Study the drawing (mm; zero at the part's minimum x, y, z) and answer. A direction names the side the tool comes from. Give positions to 0.01 mm unless a question says otherwise; leave off trailing zeros. Order: outer loops, then holes, each group sorted by start corner. A loop starts at its lowest first (then second) coordinate and runs counter-clockwise, first axis right, second up. Notation, with made-up numbers: (9.5, 43) - (23.5, 43) arc R12 ccw to (23.5, 51) - close; hole circle Ø2 at (18.5, -39). An arc over 180 degrees is marked (long way). Write each question's results on one line, items separated by ' | '. Start each with the question number.
Q1. Find section C-C on y = 48. Give the vertices of the cut face in (x, z).
Q2. A tool of negligible diameter and unlimited length cuts with its end or side. For the marked faces 4 and 5, from which of +Z, -Z, +X, -X, +Y, -Y can it reach the whole face along a straight path? Write none if from no direction.
Q3. Find section A-A on z = 48. Give the vertices of the cut face in (x, y).
Q4. Flat-ended cylindrical pins translate along their axes: P1, Ø3, axis at y = 71.5, z = 22, coming from the -X side; P2, Ø2, axis at x = 6.5, z = 35.5, coming from the +Y side; P3, Ø3, axis at x = 5, z = 37, coming from the +Y side. Find the tip coordinate at first contact, or state that the pin passes through.
Q5. For a pull along Z with two mould halves and no side action, classify the marked faces 1, 2 and 3 as +Z half, -Z half, draft (parallel to the pull), parting line (faces both ways), or undercut.
Q6. Find section B-B on x = 31. Give the vertices of the cut face in (y, z), and give its area (3 significant figures).
Q7. Find section D-D on y = 14. Give the vertices of the cut face in (x, z).
Q8. Find the intervals of material crossed by line 1 along X through (y, z) = (48, 64.5); line 2 along Z through (x, y) = (29.5, 33); line 3 along Y through (x, z) = (33.5, 20), in increasing order. Write a range as from..to.
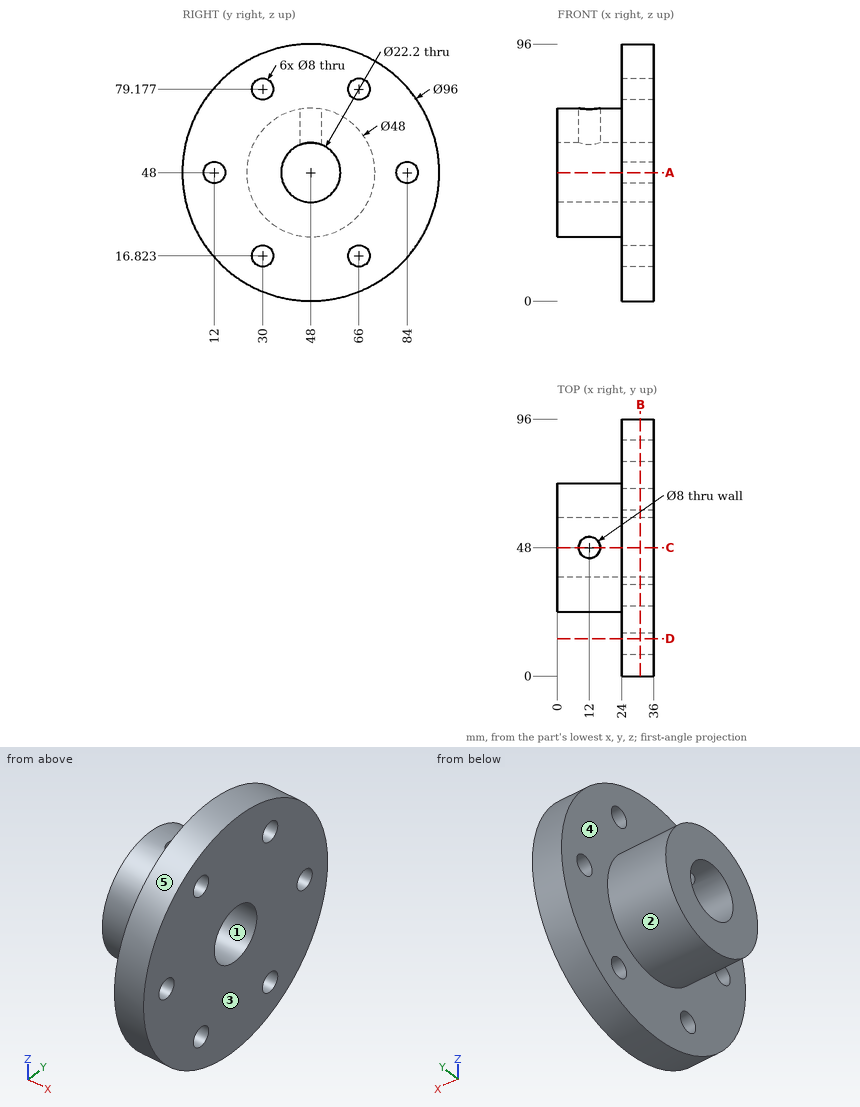
Working result:
1) outline: (0, 24) - (24, 24) - (24, 0) - (36, 0) - (36, 36.9) - (0, 36.9) - close; (0, 59.1) - (8, 59.1) - (8, 72) - (0, 72) - close; (16, 59.1) - (36, 59.1) - (36, 96) - (24, 96) - (24, 72) - (16, 72) - close
2) face 4: -X | face 5: +X, -X
3) outline: (0, 24) - (24, 24) - (24, 16) - (36, 16) - (36, 36.9) - (0, 36.9) - close; (0, 59.1) - (36, 59.1) - (36, 80) - (24, 80) - (24, 72) - (0, 72) - close; (24, 0) - (36, 0) - (36, 8) - (24, 8) - close; (24, 88) - (36, 88) - (36, 96) - (24, 96) - close
4) P1: x = 24 | P2: y = 69.07 | P3: y = 70.04
5) face 1: undercut | face 2: parting line | face 3: draft
6) outline: circle Ø96 at (48, 48); hole circle Ø8 at (12, 48); hole circle Ø8 at (30, 16.82); hole circle Ø8 at (30, 79.18); hole circle Ø22.2 at (48, 48); hole circle Ø8 at (66, 16.82); hole circle Ø8 at (66, 79.18); hole circle Ø8 at (84, 48) | area: 6,550 mm²
7) outline: (24, 14.12) - (36, 14.12) - (36, 44.54) - (24, 44.54) - close; (24, 51.46) - (36, 51.46) - (36, 81.88) - (24, 81.88) - close
8) line 1: 0..8, 16..36 | line 2: 2.4..14.18, 19.47..76.53, 81.82..93.6 | line 3: 9.01..27.57, 32.43..63.57, 68.43..86.99
